from build123d import *

# Parameters (mm, degrees)
SKETCH2_R           = 1.5
BOSS_EXTRUDE1_DEPTH = 0.97
FILLET1_R           = 3.65
FILLET2_R           = 5
SKETCH3_R           = 1.585
CUT_EXTRUDE1_DEPTH  = 29.350724858


with BuildPart() as part:
    # Sketch2 → Boss-Extrude1 (new, symmetric)
    with BuildSketch(Plane.XY):
        Polygon((-3.65, -3.65), (-3.65, -20), (3.65, -20), (3.65, -3.65), (20, -3.65), (20, 3.65), (3.65, 3.65), (3.65, 20), (-3.65, 20), (-3.65, 3.65), (-20, 3.65), (-20, -3.65), align=None)
        with Locations((-16.05, 0)):
            Circle(SKETCH2_R, mode=Mode.SUBTRACT)
        with Locations((0, -16.05)):
            Circle(SKETCH2_R, mode=Mode.SUBTRACT)
        with Locations((16.05, 0)):
            Circle(SKETCH2_R, mode=Mode.SUBTRACT)
        with Locations((0, 16.05)):
            Circle(SKETCH2_R, mode=Mode.SUBTRACT)
    extrude(amount=BOSS_EXTRUDE1_DEPTH, both=True)

    # Fillet1
    fillet1_edges = [part.edges().sort_by_distance(p)[0] for p in [
        (20, 3.65, 0),
        (20, -3.65, 0),
        (3.65, -20, 0),
        (-3.65, -20, 0),
        (-20, -3.65, 0),
        (-20, 3.65, 0),
        (3.65, 20, 0),
        (-3.65, 20, 0),
    ]]
    fillet(fillet1_edges, radius=FILLET1_R - 0.0001)  # a hair under: the kernel refuses the full size

    # Fillet2
    fillet2_edges = [part.edges().sort_by_distance(p)[0] for p in [
        (-3.65, -3.65, 0),
        (-3.65, 3.65, 0),
        (3.65, 3.65, 0),
        (3.65, -3.65, 0),
    ]]
    fillet(fillet2_edges, radius=FILLET2_R)

    # Sketch3 → Cut-Extrude1 (cut, through all)
    with BuildSketch(Plane.XY.offset(0.97)):
        Circle(SKETCH3_R)
    extrude(amount=-CUT_EXTRUDE1_DEPTH, mode=Mode.SUBTRACT)


solid = part.part
Geometry check sheet. Reference: the model listing, model coordinates, mm. A direction names the side the tool comes from. Coordinates: 2 decimals unless noted, no trailing zeros. Order: outer loops, then holes, each group sorted by start corner. A loop starts at its lowest first (then second) coordinate and runs counter-clockwise, first axis right, second up. Notation, with made-up numbers: (79.5, -34.75) - (87.5, -34.75) arc R24 cw to (87.5, 4.25) - close; hole circle Ø4 at (-4.75, 7.5). An arc over 180 degrees is marked (long way). One line per item, written item: value.
(1) Depth check by flat-ended pin: pin 1 Ø0.6 at (x, z) = (14, -0.5) entering from -Y; pin 2 Ø1 at (y, z) = (11.5, 0) entering from -X. Enter the tip coordinate at first touch or a pass-through.
Data:
pin 1: stops at y = -3.65
pin 2: stops at x = -3.65
(2) Sectioned sample at B-B (y = -13). Enter the section's corners in (x, z), and give its area (3 significant figures).
Data:
outline: (-3.65, -0.97) - (3.65, -0.97) - (3.65, 0.97) - (-3.65, 0.97) - close
area: 14.2 mm^2
(3) Release check for a two-part mould opening along X. For faces 5 (the face through (-3.65, 13, 0)), 6 (the face through (17.48, 0.45, -0.01)), 7 (the face through (3.65, -13, 0)) record: +X half, -X half, draft (parallel to the pull), parting line (faces both ways), or undercut.
Data:
face 5: -X half
face 6: undercut
face 7: +X half
(4) Access from +Z, -Z, +X, -X, +Y, -Y to the whole of each face (thin tool, end or side, straight path). Record for faces 1 (the face through (13, 3.65, 0)), 2 (the face through (1.4, -1.4, -0.97)), 3 (the face through (12, -3.65, 0)), 4 (the face through (-3.65, -12, 0)).
Data:
face 1: +Z, -Z, +X, +Y
face 2: -Z, +X, -X, +Y, -Y
face 3: +Z, -Z, +X, -Y
face 4: +Z, -Z, -X, -Y
(5) Thickness scan on probe 1 along Y at (x, z) = (0, -0.05) (3 decimals); probe 2 along X at (y, z) = (-16, 0.7). Record the ranges inside material, lowest first. Write a range as from..to.
Data:
probe 1: y = -20..-17.55, -14.55..-1.585, 1.585..14.55, 17.55..20
probe 2: x = -3.65..-1.5, 1.5..3.65
(6) Sectioned sample at A-A (z = -0.05). Count the separate pieces of the cut face and the enclosed holes in it, and give its area (3 significant figures).
Data:
separate pieces: 1
enclosed holes: 5
area: 493 mm^2
